from build123d import *

# Parameters (mm, degrees)
SKETCH_1_W          = 178
SKETCH_1_H          = 102.6
SKETCH_1_R          = 1.5
EXTRUDE_1_DEPTH     = 2
SKETCH_3_R          = 1.25
SKETCH_3_R_2        = 1.1
CUT_EXTRUDE_1_DEPTH = 103.74575417
CUT_EXTRUDE_2_DEPTH = 103.74575417
FILLET_1_R          = 3


with BuildPart() as part:
    # 草图1 → 凸台-拉伸1 (new body)
    with BuildSketch(Plane.XY):
        Rectangle(SKETCH_1_W, SKETCH_1_H)
        with Locations((-86, 25.3)):
            Circle(SKETCH_1_R, mode=Mode.SUBTRACT)
        with Locations((-86, -25.3)):
            Circle(SKETCH_1_R, mode=Mode.SUBTRACT)
        with Locations((86, 25.3)):
            Circle(SKETCH_1_R, mode=Mode.SUBTRACT)
        with Locations((86, -25.3)):
            Circle(SKETCH_1_R, mode=Mode.SUBTRACT)
    extrude(amount=EXTRUDE_1_DEPTH)

    # 草图3 → 切除-拉伸1 (cut, through all)
    with BuildSketch(Plane.XY.offset(2)):
        with Locations((-61.5, -22.5)):
            Circle(SKETCH_3_R)
        with Locations((-61.5, 22.5)):
            Circle(SKETCH_3_R)
        with Locations((61.5, -22.5)):
            Circle(SKETCH_3_R)
        with Locations((61.5, 22.5)):
            Circle(SKETCH_3_R)
        with Locations((-42.5, -22.5)):
            Circle(SKETCH_3_R_2)
        with Locations((-42.5, 22.5)):
            Circle(SKETCH_3_R_2)
        with Locations((42.5, 22.5)):
            Circle(SKETCH_3_R_2)
        with Locations((42.5, -22.5)):
            Circle(SKETCH_3_R_2)
    extrude(amount=-CUT_EXTRUDE_1_DEPTH, mode=Mode.SUBTRACT)

    # 草图4 → 切除-拉伸2 (cut, through all)
    with BuildSketch(Plane.XY.offset(2)):
        with BuildLine():
            Line((-80, -35), (-80, 35))
            ThreePointArc((-80, 35), (-73.25, 41.75), (-66.5, 35))
            Line((-66.5, 35), (-66.5, -35))
            ThreePointArc((-66.5, -35), (-73.25, -41.75), (-80, -35))
        make_face()
        with BuildLine():
            Line((80, -35), (80, 35))
            ThreePointArc((80, 35), (73.25, 41.75), (66.5, 35))
            Line((66.5, 35), (66.5, -35))
            ThreePointArc((66.5, -35), (73.25, -41.75), (80, -35))
        make_face()
        Polygon((-56.5, -24.539773754), (-56.5, 24.539773754), (-12.202964311, 0), align=None)
        Polygon((-56.5, 39.3), (0, 8), (56.5, 39.3), align=None)
        Polygon((56.5, -39.3), (-56.5, -39.3), (0, -8), align=None)
        Polygon((12.202964311, 0), (56.5, -24.539773754), (56.5, 24.539773754), align=None)
    extrude(amount=-CUT_EXTRUDE_2_DEPTH, mode=Mode.SUBTRACT)

    # 圆角1
    fillet_1_edges = [part.edges().sort_by_distance(p)[0] for p in [
        (12.202964311, 0, 1),
        (56.5, 24.539773754, 1),
        (56.5, -24.539773754, 1),
        (56.5, 39.3, 1),
        (0, 8, 1),
        (-56.5, 39.3, 1),
        (-12.202964311, 0, 1),
        (-56.5, -24.539773754, 1),
        (-56.5, 24.539773754, 1),
        (-56.5, -39.3, 1),
        (0, -8, 1),
        (56.5, -39.3, 1),
    ]]
    fillet(fillet_1_edges, radius=FILLET_1_R)


solid = part.part
Design review of the part built by this model. Coordinates are the model's own, in mm. A direction names the side the tool comes from. Coordinates: 2 decimals unless noted, no trailing zeros. Order: outer loops, then holes, each group sorted by start corner. A loop starts at its lowest first (then second) coordinate and runs counter-clockwise, first axis right, second up.
Item 1: Take a section at D-D, the plane x = 77. Write out the cut boundary in (y, z), then the cut area to 4 significant figures.
Item 2: For pin 1 Ø8 at (x, y) = (-30.5, 29) entering from -Z, flat-tipped, find the tip position at first contact; note if it passes through.
Item 3: For line 1 (Y direction, x = 61.5, z = 1); line 2 (Y direction, x = -86, z = 0.85); line 3 (X direction, y = 12, z = 1.45), list the stretches that pass through material, from the lowest coordinate up.
Item 4: For faces 1 (the flat face through (23.59, -21.07, 1.01)), 2 (the flat face through (-1, 1, 0)), list the 3-axis set-ups (+Z, -Z, +X, -X, +Y, -Y) from which the entire face can be reached by the end or side of a thin tool; tool diameter is ignored.
Item 5: Take a section at B-B, the plane x = 33.5. Write out the cut boundary in (y, z).
Item 6: Take a section at A-A, the plane x = -73.25. Write out the cut boundary in (y, z).
Item 7: The part is to be moulded in two halves that separate along Y. For faces 3 (the cylindrical face through (-73.1, -41.75, 1.01)), 4 (the flat face through (-1, 1, 2)), say which applies: pulls with the +Y half, pulls with the -Y half, needs draft (parallel to the pull), parting line crosses it, or undercut.
Item 8: Take a section at C-C, the plane z = 1.55. Count the separate pieces of the cut face and the enclosed holes in it, then the cut area to 3 significant figures.
The answers:
1. outline: (-51.3, 0) - (-40.61, 0) - (-40.61, 2) - (-51.3, 2) - close; (40.61, 0) - (51.3, 0) - (51.3, 2) - (40.61, 2) - close
1. area: 42.75 mm2
2. pin 1: stops at z = 0
3. line 1: y = -51.3 to -23.75, -21.25 to 21.25, 23.75 to 51.3
3. line 2: y = -51.3 to -26.8, -23.8 to 23.8, 26.8 to 51.3
3. line 3: x = -89 to -80, -66.5 to -56.5, -33.86 to -7.22, 7.22 to 33.86, 56.5 to 66.5, 80 to 89
4. face 1: +Z, -Z
4. face 2: -Z, +X, -X, +Y, -Y
5. outline: (-51.3, 0) - (-39.3, 0) - (-39.3, 2) - (-51.3, 2) - close; (-26.56, 0) - (-11.8, 0) - (-11.8, 2) - (-26.56, 2) - close; (11.8, 0) - (26.56, 0) - (26.56, 2) - (11.8, 2) - close; (39.3, 0) - (51.3, 0) - (51.3, 2) - (39.3, 2) - close
6. outline: (-51.3, 0) - (-41.75, 0) - (-41.75, 2) - (-51.3, 2) - close; (41.75, 0) - (51.3, 0) - (51.3, 2) - (41.75, 2) - close
7. face 3: undercut
7. face 4: needs draft
8. separate pieces: 1
8. enclosed holes: 18
8. area: 10,400 mm2
